```python
from build123d import *

# Parameters (mm, degrees)
CYLINDER002_R        = 0.5
CYLINDER002_DEPTH    = 0.5
CYLINDER003_R        = 0.2
CYLINDER003_DEPTH    = 10
FUSION002_ROLL_ANGLE = 90
CYLINDER_R           = 0.5
CYLINDER_DEPTH       = 0.5
CYLINDER001_R        = 0.2
CYLINDER001_DEPTH    = 10
FUSION001_ROLL_ANGLE = 90
PAD_DEPTH            = 120
PAD002_DEPTH         = 1.4
PAD001_DEPTH         = 1.4


with BuildPart() as cylinder002:
    # Cylinder002 → Cylinder002 (new body)
    with BuildSketch(Plane(origin=(0, 3, 0), x_dir=(1, 0, 0), z_dir=(0, 0, 1))):
        Circle(CYLINDER002_R)
    extrude(amount=CYLINDER002_DEPTH)


with BuildPart() as screwhole2:
    # Cylinder003 → Cylinder003 (new body)
    with BuildSketch(Plane(origin=(0, 3, 0), x_dir=(1, 0, 0), z_dir=(0, 0, 1))):
        Circle(CYLINDER003_R)
    extrude(amount=CYLINDER003_DEPTH)

    # Fusion002: union Cylinder002
    add(cylinder002.part)


with BuildPart() as screwhole2_1:
    # Fusion002 roll: moved
    add(screwhole2.part.rotate(Axis((0, 0, 0), (1, 0, 0)), FUSION002_ROLL_ANGLE))


with BuildPart() as screwhole2_2:
    # Fusion002 placement: moved
    add(screwhole2_1.part.moved(Location((10, 1, 115.5))))


with BuildPart() as cylinder:
    # Cylinder → Cylinder (new body)
    with BuildSketch(Plane(origin=(0, 3, 0), x_dir=(1, 0, 0), z_dir=(0, 0, 1))):
        Circle(CYLINDER_R)
    extrude(amount=CYLINDER_DEPTH)


with BuildPart() as screws:
    # Cylinder001 → Cylinder001 (new body)
    with BuildSketch(Plane(origin=(0, 3, 0), x_dir=(1, 0, 0), z_dir=(0, 0, 1))):
        Circle(CYLINDER001_R)
    extrude(amount=CYLINDER001_DEPTH)

    # Fusion001: union Cylinder
    add(cylinder.part)


with BuildPart() as screws_1:
    # Fusion001 roll: moved
    add(screws.part.rotate(Axis((0, 0, 0), (1, 0, 0)), FUSION001_ROLL_ANGLE))


with BuildPart() as screws_2:
    # Fusion001 placement: moved
    add(screws_1.part.moved(Location((10, 1, -1.5))))

    # Fusion003: union screwhole2
    add(screwhole2_2.part)


with BuildPart() as obj1:
    # Sketch → Pad (new body)
    with BuildSketch(Plane.XY):
        Polygon((-1, 1), (21, 1), (21, -24.7), (20, -24.7), (20, 0), (11.9, 0), (11.9, -0.5), (8.1, -0.5), (8.1, 0), (0, 0), (0, -24.7), (-1, -24.7), align=None)
    extrude(amount=PAD_DEPTH)


with BuildPart() as upper_slide:
    # Sketch002 → Pad002 (new body)
    with BuildSketch(Plane.XY.offset(118.6)):
        Polygon((0, 0), (20, 0), (20, -19), (18.6, -19), (18.6, -0.5), (1.4, -0.5), (1.4, -19), (0, -19), align=None)
    extrude(amount=PAD002_DEPTH)


with BuildPart() as obj2:
    # Sketch001 → Pad001 (new body)
    with BuildSketch(Plane.XY):
        Polygon((0, 0), (20, 0), (20, -19), (18.6, -19), (18.6, -0.5), (1.4, -0.5), (1.4, -19), (0, -19), align=None)
    extrude(amount=PAD001_DEPTH)

    # Fusion: union obj1, upper_slide
    add(obj1.part)
    add(upper_slide.part)

    # Cut: cut screws
    add(screws_2.part, mode=Mode.SUBTRACT)


solid = obj2.part
```
Can you work these out from the model? Positions are in its coordinate system, mm. A direction names the side the tool comes from. Coordinates: 2 decimals unless noted, no trailing zeros. Loops run counter-clockwise (first coordinate to the right, second up) from the corner with the lowest first, then second, coordinate; pieces in that order, holes last. Notation, with made-up numbers: (-13.75, 78) - (32.25, 78) arc R20 cw to (32.25, 104) - close; hole circle Ø5 at (77.5, -29.5). An arc over 180 degrees is marked (long way). Answer as CSV lines item,"result". Start each with the question number.
1) I need wall thicknesses on line 1 (Z direction, x = 10, y = 0.6); line 2 (Z direction, x = 10, y = -0.2); line 3 (X direction, y = -0.3, z = 118.5). Which ranges of each line are inside material? Lowest first, please. Write a range as from..to.
2) For pin 1 (9 mm diameter, centred on x = 14.5, z = 74.5, fed in from -Y); pin 2 (3 mm diameter, centred on x = 9.5, y = -3.5, fed in from +Z), each with a flat end and sliding along its axis, tell me the tip position at first contact or that it passes through.
3) Suppose I cut it at A-A (x = 16.25). Please give me the cut outline in (y, z).
4) Which directions (+Z, -Z, +X, -X, +Y, -Y) give clear straight access to the entire face, cutting with the end or side of a thin tool? Please do faces 1 (the flat face through (1, -8, 1.4)), 2 (the flat face through (9, -0.5, 60)), 3 (the flat face through (10.1, 0.6, 120)).
5) Thinking about a two-plate mould opening in Z: for faces 4 (the flat face through (10, 1, 59)), 5 (the flat face through (16, 0, 59)), 6 (the flat face through (10.1, 0.6, 0)), which applies, pulls with the +Z half, pulls with the -Z half, needs draft (parallel to the pull), parting line crosses it, or undercut?
6) Suppose I cut it at C-C (z = 91). Please give me the cut outline in (x, y), plus the area to 3 significant figures.
7) Suppose I cut it at B-B (y = -14). Please give me the cut outline in (x, z).
Check result:
1,line 1,"z = 0..1, 2..118, 119..120"
1,line 2,"z = 0..1.3, 1.7..118.3, 118.7..120"
1,line 3,"x = -1..0, 8.1..9.8, 10.2..11.9, 20..21"
2,pin 1,"stops at y = -0.5"
2,pin 2,"passes through"
3,outline,"(-0.5, 0) - (1, 0) - (1, 120) - (-0.5, 120) - (-0.5, 118.6) - (0, 118.6) - (0, 1.4) - (-0.5, 1.4) - close"
4,face 1,"-Y"
4,face 2,"+Z, -Z, -Y"
4,face 3,"+Z, +X, -X, +Y, -Y"
5,face 4,"needs draft"
5,face 5,"undercut"
5,face 6,"pulls with the -Z half"
6,outline,"(-1, -24.7) - (0, -24.7) - (0, 0) - (8.1, 0) - (8.1, -0.5) - (11.9, -0.5) - (11.9, 0) - (20, 0) - (20, -24.7) - (21, -24.7) - (21, 1) - (-1, 1) - close"
6,area,"73.3 mm²"
7,outline,"(-1, 0) - (1.4, 0) - (1.4, 1.4) - (0, 1.4) - (0, 118.6) - (1.4, 118.6) - (1.4, 120) - (-1, 120) - close; (18.6, 0) - (21, 0) - (21, 120) - (18.6, 120) - (18.6, 118.6) - (20, 118.6) - (20, 1.4) - (18.6, 1.4) - close"
